```python
from build123d import *

# Parameters (mm, degrees)
ESQUISSE2_W             = 44
ESQUISSE2_H             = 44
ENL_V_MAT_EXTRU_1_DEPTH = 38
ESQUISSE3_W             = 3.666666666
ESQUISSE3_H             = 3.666666666
ENL_V_MAT_EXTRU_2_DEPTH = 0.044


with BuildPart() as part:
    # Esquisse1 → Révolution1 (revolve)
    with BuildSketch(Plane.XY, mode=Mode.PRIVATE) as r_volution1_sk:
        with BuildLine():
            Line((0, 8.105), (0, 2.73))
            ThreePointArc((0, 2.73), (0.21381205, 2.21381205), (0.73, 2))
            Line((0.73, 2), (32, 2))
            Line((32, 2), (32, 9.3))
            ThreePointArc((32, 9.3), (34.7551415, 8.301392936), (36.23060683, 5.76939317))
            ThreePointArc((36.23060683, 5.76939317), (36.921370264, 4.938703552), (38, 5))
            ThreePointArc((38, 5), (36.242640687, 9.242640687), (32, 11))
            Line((32, 11), (31, 11))
            Line((31, 11), (27.333333333, 14.666666667))
            Line((27.333333333, 14.666666667), (21, 14.666666667))
            Line((21, 14.666666667), (21, 9.3))
            Line((21, 9.3), (13, 9.3))
            Line((13, 9.3), (13, 14.666666667))
            Line((13, 14.666666667), (8, 14.666666667))
            Line((8, 14.666666667), (8, 8.835))
            Line((8, 8.835), (6.4, 8.835))
            Line((6.4, 8.835), (5.594596374, 9.3))
            Line((5.594596374, 9.3), (0.8, 9.3))
            Line((0.8, 9.3), (0.8, 8.835))
            Line((0.8, 8.835), (0.73, 8.835))
            ThreePointArc((0.73, 8.835), (0.21381205, 8.62118795), (0, 8.105))
        make_face()
    revolve(r_volution1_sk.sketch.rotate(Axis((38, 0, 0), (-1, 0, 0)), 90), axis=Axis((38, 0, 0), (-1, 0, 0)))

    # Esquisse2 → Enlèv. mat.-Extru.1 (cut)
    with BuildSketch(Plane(origin=(8, 0, 0), x_dir=(0, 0, -1), z_dir=(1, 0, 0))):
        Rectangle(ESQUISSE2_W, ESQUISSE2_H)
        with BuildLine():
            Line((-11, 5.276362383), (-11, -5.276362383))
            ThreePointArc((-11, -5.276362383), (-10.565509926, -6.1), (-10.069463864, -6.88809825))
            Line((-10.069463864, -6.88809825), (-0.930536136, -12.164460633))
            ThreePointArc((-0.930536136, -12.164460633), (0, -12.2), (0.930536136, -12.164460633))
            Line((0.930536136, -12.164460633), (10.069463864, -6.88809825))
            ThreePointArc((10.069463864, -6.88809825), (10.565509926, -6.1), (11, -5.276362383))
            Line((11, -5.276362383), (11, 5.276362383))
            ThreePointArc((11, 5.276362383), (10.565509926, 6.1), (10.069463864, 6.88809825))
            Line((10.069463864, 6.88809825), (0.930536136, 12.164460633))
            ThreePointArc((0.930536136, 12.164460633), (0, 12.2), (-0.930536136, 12.164460633))
            Line((-0.930536136, 12.164460633), (-10.069463864, 6.88809825))
            ThreePointArc((-10.069463864, 6.88809825), (-10.565509926, 6.1), (-11, 5.276362383))
        make_face(mode=Mode.SUBTRACT)
    extrude(amount=ENL_V_MAT_EXTRU_1_DEPTH, mode=Mode.SUBTRACT)

    # Esquisse3 → Enlèv. mat.-Extru.2 (cut)
    with BuildSketch(Plane.XY.offset(11)):
        with Locations((10.5, 0)):
            Rectangle(ESQUISSE3_W, ESQUISSE3_H)
        with BuildLine():
            Line((9.390432265, -1.243638701), (9.465872252, -1.139804467))
            ThreePointArc((9.465872252, -1.139804467), (10.23876211, -0.359563109), (9.735544583, -1.335732884))
            Line((9.735544583, -1.335732884), (9.660104596, -1.439567118))
            ThreePointArc((9.660104596, -1.439567118), (10.5, -1.666666667), (11.339895404, -1.439567118))
            Line((11.339895404, -1.439567118), (11.264455417, -1.335732884))
            ThreePointArc((11.264455417, -1.335732884), (10.76123789, -0.359563109), (11.534127748, -1.139804467))
            Line((11.534127748, -1.139804467), (11.609567735, -1.243638701))
            ThreePointArc((11.609567735, -1.243638701), (12.085094194, -0.515028324), (12.128651642, 0.353937293))
            Line((12.128651642, 0.353937293), (12.006587179, 0.314276144))
            ThreePointArc((12.006587179, 0.314276144), (10.922691785, 0.137340886), (11.903581514, 0.631294983))
            Line((11.903581514, 0.631294983), (12.025645977, 0.670956131))
            ThreePointArc((12.025645977, 0.670956131), (11.479642087, 1.348361657), (10.666666667, 1.658312395))
            Line((10.666666667, 1.658312395), (10.666666667, 1.529966223))
            ThreePointArc((10.666666667, 1.529966223), (10.5, 0.444444444), (10.333333333, 1.529966223))
            Line((10.333333333, 1.529966223), (10.333333333, 1.658312395))
            ThreePointArc((10.333333333, 1.658312395), (9.520357913, 1.348361657), (8.974354023, 0.670956131))
            Line((8.974354023, 0.670956131), (9.096418486, 0.631294983))
            ThreePointArc((9.096418486, 0.631294983), (10.077308215, 0.137340886), (8.993412821, 0.314276144))
            Line((8.993412821, 0.314276144), (8.871348358, 0.353937293))
            ThreePointArc((8.871348358, 0.353937293), (8.914905806, -0.515028324), (9.390432265, -1.243638701))
        make_face(mode=Mode.SUBTRACT)
    extrude(amount=-ENL_V_MAT_EXTRU_2_DEPTH, mode=Mode.SUBTRACT)


solid = part.part
```
Build history of the part. All positions in model axes, mm. A direction names the side the tool comes from. Give positions to 0.01 mm unless a question says otherwise; leave off trailing zeros. Loops run counter-clockwise (first coordinate to the right, second up) from the corner with the lowest first, then second, coordinate; pieces in that order, holes last.
Item 1: Which spindle directions (+Z, -Z, +X, -X, +Y, -Y) get a long thin tool onto all of the face, cutting with end or side? Do faces 1 (the face through (25.3, 12.2, 0)), 2 (the face through (21, 8.1, 4.9)). Say none if no direction does.
Answers follow:
face 1: +X, -X, +Y
face 2: none
Item 2: Slice it at A-A, the plane x = 28.5. List the corners of the cut face in (y, z), and give its area (3 significant figures).
Answers follow:
outline: (-12.16, -0.93) - (-6.89, -10.07) arc R12.2 ccw to (-5.28, -11) - (5.28, -11) arc R12.2 ccw to (6.89, -10.07) - (12.16, -0.93) arc R12.2 ccw to (12.16, 0.93) - (6.89, 10.07) arc R12.2 ccw to (5.28, 11) - (-5.28, 11) arc R12.2 ccw to (-6.89, 10.07) - (-12.16, 0.93) arc R12.2 ccw to start; hole circle Ø4 at (0, 0)
area: 404 mm2
Item 3: Pull direction Y, two halves, no side cores. Call faces 3 (the face through (8.2, 0.1, 11)), 4 (the face through (10.46, 9.56, 5.44)), 5 (the face through (25.93, -9.56, -5.44)), 6 (the face through (10.5, 0.8, 10.956)): released by +Y, released by -Y, zero draft, split by the parting line, or undercut.
Answers follow:
face 3: zero draft
face 4: released by +Y
face 5: released by -Y
face 6: undercut
Item 4: Flat gauge pins, fed straight in: pin 1 (1 mm diameter, centred on x = 15, y = -8, fed in from +Z); pin 2 (6 mm diameter, centred on x = 15.5, y = 7, fed in from -Z); pin 3 (3 mm diameter, centred on x = 9.5, z = 7.5, fed in from +Y). Where does each tip first touch, or does it go through?
Answers follow:
pin 1: stops at z = 5.5
pin 2: stops at z = -10.97
pin 3: stops at y = 9.24
Item 5: Drill centre lines: line 1 (Y direction, x = 14.5, z = 0); line 2 (X direction, y = 4.25, z = -4.5); line 3 (Z direction, x = 27.5, y = 0.75). Where is each one in solid material? Low to high.
Answers follow:
line 1: y = -9.3 to -2, 2 to 9.3
line 2: x = 0 to 32, 36.13 to 37.88
line 3: z = -11 to -1.85, 1.85 to 11
Item 6: Slice it at B-B, the plane x = 18.5. List the corners of the cut face in (y, z).
Answers follow:
outline: circle Ø18.6 at (0, 0); hole circle Ø4 at (0, 0)
